Work out the finished part from the listing and answer in its coordinate system (mm). Face numbers are marked on the shaded views. A direction names the side the tool comes from. Round coordinates to 2 decimals unless told otherwise and drop trailing zeros. Loops run counter-clockwise (first coordinate to the right, second up) from the corner with the lowest first, then second, coordinate; pieces in that order, holes last. Notation, with made-up numbers: M 37,44.25 L 46,44.25 A24 cw 46,67.25 Z; hole C 46,-2 d6. An arc over 180 degrees is marked long. One line per item, written item: value.
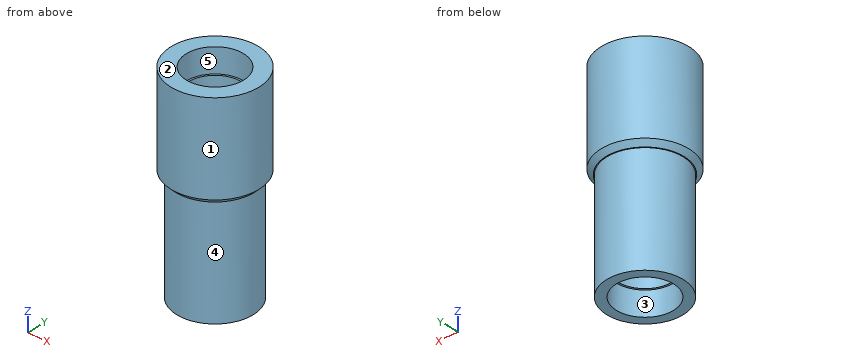
```python
from build123d import *

# Parameters (mm, degrees)
SKETCH1_R          = 4.5974
EXTRUDE1_DEPTH     = 21.463
SKETCH3_R          = 2.794
CUT_EXTRUDE2_DEPTH = 23.426157551
SKETCH4_R          = 2.9972
CUT_EXTRUDE3_DEPTH = 2.54
SKETCH5_OUTSIDE_W  = 16.212
SKETCH5_OUTSIDE_H  = 16.212
SKETCH5_OUTSIDE_R  = 4.0005
CUT_EXTRUDE4_DEPTH = 11.43
CUT_EXTRUDE5_START = -2.54
SKETCH6_R          = 2.9972
CUT_EXTRUDE5_DEPTH = 2.54
CHAMFER1_SIZE      = 0.508


with BuildPart() as part:
    # Sketch1 → Extrude1 (new body)
    with BuildSketch(Plane.XY):
        Circle(SKETCH1_R)
    extrude(amount=EXTRUDE1_DEPTH)

    # Sketch3 → Cut-Extrude2 (cut, through all)
    with BuildSketch(Plane.XY.offset(21.463)):
        Circle(SKETCH3_R)
    extrude(amount=-CUT_EXTRUDE2_DEPTH, mode=Mode.SUBTRACT)

    # Sketch4 → Cut-Extrude3 (cut)
    with BuildSketch(Plane.XY.offset(21.463)):
        Circle(SKETCH4_R)
    extrude(amount=-CUT_EXTRUDE3_DEPTH, mode=Mode.SUBTRACT)

    # Sketch5 outside → Cut-Extrude4 (cut)
    with BuildSketch(Plane(origin=(0, 0, 0), x_dir=(-1, 0, 0), z_dir=(0, 0, -1))):
        Rectangle(SKETCH5_OUTSIDE_W, SKETCH5_OUTSIDE_H)
        Circle(SKETCH5_OUTSIDE_R, mode=Mode.SUBTRACT)
    extrude(amount=-CUT_EXTRUDE4_DEPTH, mode=Mode.SUBTRACT)

    # Sketch6 → Cut-Extrude5 (cut)
    with BuildSketch(Plane(origin=(0, 0, 0), x_dir=(-1, 0, 0), z_dir=(0, 0, -1)).offset(CUT_EXTRUDE5_START)):
        with Locations(Location((0, 0, 0), (0, 0, 180))):
            Circle(SKETCH6_R)
    extrude(amount=CUT_EXTRUDE5_DEPTH, mode=Mode.SUBTRACT)

    # Chamfer1
    chamfer1_edges = [part.edges().sort_by_distance(p)[0] for p in [
        (-4.5974, 0, 11.43),
    ]]
    chamfer(chamfer1_edges, length=CHAMFER1_SIZE)


solid = part.part
```
1) Find section D-D (z = 19.75). Give the vertices of the cut face in (x, y).
Check values:
outline: C 0,0 d9.19; hole C 0,0 d5.99
2) The mould has two halves that part along X. Classify the marked faces 1, 2 and 3: +X half, -X half, draft (parallel to the pull), parting line (faces both ways), or undercut.
Check values:
face 1: parting line
face 2: draft
face 3: undercut
3) Find section C-C (z = 3). Give the vertices of the cut face in (x, y), then the cut area to 3 significant figures.
Check values:
outline: C 0,0 d8; hole C 0,0 d5.59
area: 25.8 mm2
4) For the marked faces 4 and 5, determine the directions among +Z, -Z, +X, -X, +Y, -Y from which every point of the face is accessible in a straight line to the end or side of a thin tool.
Check values:
face 4: -Z
face 5: +Z
5) Find section A-A (x = 0). Give the vertices of the cut face in (y, z), then the cut area to 3 significant figures.
Check values:
outline: M -4.6,11.94 L -4.09,11.43 L -4,11.43 L -4,0 L -3,0 L -3,2.54 L -2.79,2.54 L -2.79,18.92 L -3,18.92 L -3,21.46 L -4.6,21.46 Z; M 2.79,2.54 L 3,2.54 L 3,0 L 4,0 L 4,11.43 L 4.09,11.43 L 4.6,11.94 L 4.6,21.46 L 3,21.46 L 3,18.92 L 2.79,18.92 Z
area: 61.4 mm2
6) Each of these flat-tipped pins is pushed along its axis until it touches: pin 1 (5 mm diameter, centred on x = 2, z = 5.5, fed in from -Y); pin 2 (1.5 mm diameter, centred on x = -3, z = 4, fed in from -Y); pin 3 (1 mm diameter, centred on x = -1, z = 16, fed in from -Y). Where does it stop, or does it pass through?
Check values:
pin 1: y = -4
pin 2: y = -3.31
pin 3: y = -4.57
7) Find the intervals of material crossed by probe 1 along Y at (x, z) = (0, 1.4); probe 2 along Y at (x, z) = (0, 20.9); probe 3 along X at (y, z) = (-1.5, 9.5), in increasing order. Write a range as from..to.
Check values:
probe 1: -4..-3, 3..4
probe 2: -4.6..-3, 3..4.6
probe 3: -3.71..-2.36, 2.36..3.71
